from build123d import *

# Parameters (mm, degrees)
CROQUIS1_R              = 2.5
SALIENTE_EXTRUIR1_DEPTH = 5
REDONDEO1_R             = 2


with BuildPart() as part:
    # Croquis1 → Saliente-Extruir1 (new body)
    # profile 1 of 4: a face of its own
    with BuildSketch(Plane(origin=(0, 0, 0), x_dir=(1, 0, 0), z_dir=(0, 1, 0))):
        Polygon((0, 79), (0, 91), (15, 91), (15, 85), (79, 85), (79, 91), (91, 91), (91, 79), (85, 79), (85, 15), (91, 15), (91, 0), (79, 0), (79, 79), align=None)
        with Locations(Location((85, 85, 0), (0, 0, 270))):
            Circle(CROQUIS1_R, mode=Mode.SUBTRACT)
    # profile 2 of 4: a face of its own
    with BuildSketch(Plane(origin=(0, 0, 0), x_dir=(1, 0, 0), z_dir=(0, 1, 0))):
        Polygon((79, 0), (91, 0), (91, -15), (85, -15), (85, -79), (91, -79), (91, -91), (79, -91), (79, -85), (15, -85), (15, -91), (0, -91), (0, -79), (79, -79), align=None)
        with Locations(Location((85, -85, 0), (0, 0, 270))):
            Circle(CROQUIS1_R, mode=Mode.SUBTRACT)
    # profile 3 of 4: a face of its own
    with BuildSketch(Plane(origin=(0, 0, 0), x_dir=(1, 0, 0), z_dir=(0, 1, 0))):
        Polygon((0, -79), (0, -91), (-15, -91), (-15, -85), (-79, -85), (-79, -91), (-91, -91), (-91, -79), (-85, -79), (-85, -15), (-91, -15), (-91, 0), (-79, 0), (-79, -79), align=None)
        with Locations(Location((-85, -85, 0), (0, 0, 270))):
            Circle(CROQUIS1_R, mode=Mode.SUBTRACT)
    # profile 4 of 4: a face of its own
    with BuildSketch(Plane(origin=(0, 0, 0), x_dir=(1, 0, 0), z_dir=(0, 1, 0))):
        Polygon((0, 79), (-79, 79), (-79, 0), (-91, 0), (-91, 15), (-85, 15), (-85, 79), (-91, 79), (-91, 91), (-79, 91), (-79, 85), (-15, 85), (-15, 91), (0, 91), align=None)
        with Locations(Location((-85, 85, 0), (0, 0, 270))):
            Circle(CROQUIS1_R, mode=Mode.SUBTRACT)
    extrude(amount=SALIENTE_EXTRUIR1_DEPTH)

    # Redondeo1
    redondeo1_edges = [part.edges().sort_by_distance(p)[0] for p in [
        (79, 2.5, -85),
        (85, 2.5, -79),
        (85, 2.5, 79),
        (79, 2.5, 85),
        (-79, 2.5, 85),
        (-85, 2.5, 79),
        (-85, 2.5, -79),
        (-79, 2.5, -85),
    ]]
    fillet(redondeo1_edges, radius=REDONDEO1_R)


solid = part.part
Design review of the part built by this model. Coordinates are the model's own, in mm. A direction names the side the tool comes from. Give positions to 0.01 mm unless a question says otherwise; leave off trailing zeros. Loops run counter-clockwise (first coordinate to the right, second up) from the corner with the lowest first, then second, coordinate; pieces in that order, holes last. Notation, with made-up numbers: M -24,81 L 6,81 A22 cw 6,91 Z; hole C 67.25,-26 d11. An arc over 180 degrees is marked long. Write item = value, one per line.
Q1. We need section A-A (x = 41). Give the boundary of the cut face in (y, z).
Output values:
outline = M 0,-85 L 5,-85 L 5,-79 L 0,-79 Z; M 0,79 L 5,79 L 5,85 L 0,85 Z
Q2. Draft analysis for pull direction X (two halves, no side actions). For faces 1 (the flat face through (-85, 2, -46)), 2 (the flat face through (88, 2, -15)), 3 (the cylindrical face through (87.48, 2.46, -85.33)), state which applies: +X half, -X half, draft (parallel to the pull), parting line (faces both ways), or undercut.
Output values:
face_1 = -X half
face_2 = draft
face_3 = undercut
Q3. For faces 4 (the flat face through (-89, 2, -79)), 5 (the flat face through (-79, 2, -1)), 6 (the flat face through (-79, 2, 89)), 7 (the flat face through (85, 2, -46)), 8 (the flat face through (-46, 2, -85)), list the 3-axis set-ups (+Z, -Z, +X, -X, +Y, -Y) from which the entire face can be reached by the end or side of a thin tool; tool diameter is ignored.
Output values:
face_4 = -X, +Y, -Y
face_5 = +Y, -Y
face_6 = +Z, +Y, -Y
face_7 = +X, +Y, -Y
face_8 = -Z, +Y, -Y
Q4. We need section B-B (z = 51.5). Give the boundary of the cut face in (x, y), plus the area to 3 significant figures.
Output values:
outline = M -85,0 L -79,0 L -79,5 L -85,5 Z; M 79,0 L 85,0 L 85,5 L 79,5 Z
area = 60.0 mm^2
Q5. Insertion check: pin 1 (2.5 mm diameter, centred on y = 3.5, z = -49, fed in from -X); pin 2 (1.5 mm diameter, centred on y = 2.5, z = -34.5, fed in from +X); pin 3 (1 mm diameter, centred on x = 24.5, y = 4, fed in from +Z); pin 4 (6.5 mm diameter, centred on x = 85, z = 85, fed in from +Y). Each pin has a flat end and moves straight along its axis. Give the tip position at first contact, or say it passes through.
Output values:
pin_1 = -85
pin_2 = 85
pin_3 = 85
pin_4 = 5
Q6. To check wall thickness, follow line 1 (X direction, y = 0.55, z = 56); line 2 (X direction, y = 2.9, z = 2). State the ranges of each line that lie inside material, in increasing order. Write a range as [from, to].
Output values:
line_1 = [-85, -79], [79, 85]
line_2 = [-91, -79], [79, 91]
Q7. We need section C-C (y = 1.95). Count the separate pieces of the cut face and the enclosed holes in it, plus the area to 3 significant figures.
Output values:
separate_pieces = 1
enclosed_holes = 5
area = 5,020 mm^2
